Input: part model. Units: mm. Frame: model coordinates. Coordinates: 2 decimals unless noted, no trailing zeros. Loops run counter-clockwise (first coordinate to the right, second up) from the corner with the lowest first, then second, coordinate; pieces in that order, holes last. Notation, with made-up numbers: (45.25, -25) -> (93.25, -25) arc R26 cw to (93.25, -1) -> close; hole circle Ø10 at (66.25, 25). An arc over 180 degrees is marked (long way). Put each result on its own line as item: value. Start each with the question number.
1) Cut plane A-A (x = 29.5). Return the cut outline in (y, z).
2) Material intervals for L1, parallel to X at y = 8.5, z = 0.1; L2, parallel to X at y = 17.75, z = 0.3; L3, parallel to X at y = 11.25, z = 0.2, sorted ascending.
3) Cut plane B-B (z = 0.3). State how many separate pieces and enclosed holes the cut face has, plus the area to 3 significant figures.
4) Contact query for a flat-ended pin moving along its axis: P1, Ø2.5, axis at x = 29.63, y = 17.86, coming from the +Z side. Output: stop coordinate, or through.
from build123d import *

# Parameters (mm, degrees)
ESBO_O1_W                = 34.00000312
ESBO_O1_H                = 21.00000372
ESBO_O1_R                = 0.4499991
RESSALTO_EXTRUS_O1_DEPTH = 0.41148
ESBO_O2_R                = 1.625
CORTE_EXTRUS_O1_DEPTH    = 1.41148


with BuildPart() as part:
    # Esboço1 → Ressalto-extrusão1 (new body)
    with BuildSketch(Plane.XY.offset(0.41148)):
        with Locations((17.00001426, 10.50001456)):
            Rectangle(ESBO_O1_W, ESBO_O1_H)
        with Locations((29.409885994, 11.411813558)):
            Circle(ESBO_O1_R, mode=Mode.SUBTRACT)
        with Locations((29.409885994, 8.871813558)):
            Circle(ESBO_O1_R, mode=Mode.SUBTRACT)
        with Locations((29.409885994, 13.951813558)):
            Circle(ESBO_O1_R, mode=Mode.SUBTRACT)
        with Locations((29.409885994, 6.331813558)):
            Circle(ESBO_O1_R, mode=Mode.SUBTRACT)
        with Locations((4.030717622, 3.815479677)):
            Circle(ESBO_O1_R, mode=Mode.SUBTRACT)
        with Locations((4.030717622, 13.975479677)):
            Circle(ESBO_O1_R, mode=Mode.SUBTRACT)
        with Locations((4.030717622, 11.435479677)):
            Circle(ESBO_O1_R, mode=Mode.SUBTRACT)
        with Locations((4.030717622, 16.515479677)):
            Circle(ESBO_O1_R, mode=Mode.SUBTRACT)
        with Locations((4.030717622, 6.355479677)):
            Circle(ESBO_O1_R, mode=Mode.SUBTRACT)
        with Locations((4.030717622, 8.895479677)):
            Circle(ESBO_O1_R, mode=Mode.SUBTRACT)
    extrude(amount=-RESSALTO_EXTRUS_O1_DEPTH)

    # Esboço2 → Corte-extrusão1 (cut, through all)
    with BuildSketch(Plane.XY.offset(0.41148)):
        with Locations((29.625048643, 17.858037309)):
            Circle(ESBO_O2_R)
        with Locations((29.625048643, 2.658236219)):
            Circle(ESBO_O2_R)
    extrude(amount=-CORTE_EXTRUS_O1_DEPTH, mode=Mode.SUBTRACT)


solid = part.part
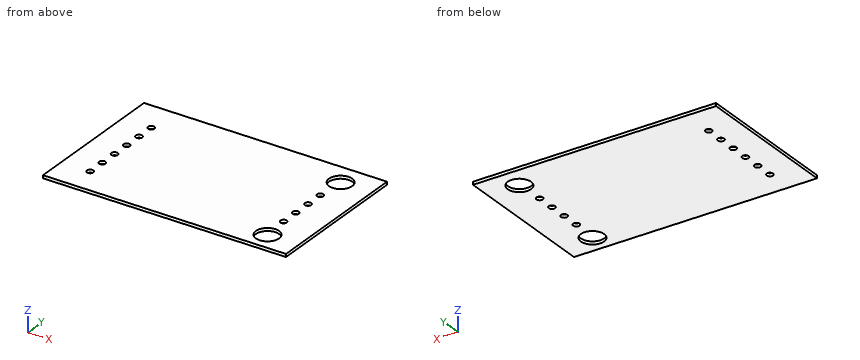
Results found:
1. outline: (0, 0) -> (1.04, 0) -> (1.04, 0.41) -> (0, 0.41) -> close; (4.28, 0) -> (5.89, 0) -> (5.89, 0.41) -> (4.28, 0.41) -> close; (6.77, 0) -> (8.43, 0) -> (8.43, 0.41) -> (6.77, 0.41) -> close; (9.31, 0) -> (10.97, 0) -> (10.97, 0.41) -> (9.31, 0.41) -> close; (11.85, 0) -> (13.51, 0) -> (13.51, 0.41) -> (11.85, 0.41) -> close; (14.39, 0) -> (16.24, 0) -> (16.24, 0.41) -> (14.39, 0.41) -> close; (19.48, 0) -> (21, 0) -> (21, 0.41) -> (19.48, 0.41) -> close
2. L1: x = 0 to 3.82, 4.25 to 29.16, 29.66 to 34
2. L2: x = 0 to 28, 31.25 to 34
2. L3: x = 0 to 3.62, 4.44 to 28.99, 29.83 to 34
3. separate pieces: 1
3. enclosed holes: 12
3. area: 691 mm2
4. P1: passes through
